```python
from build123d import *

# Parameters (mm, degrees)
SKETCH2_W           = 415
SKETCH2_H           = 210
BOSS_EXTRUDE1_DEPTH = 3
SKETCH3_W           = 415
SKETCH3_H           = 210
BOSS_EXTRUDE2_DEPTH = 3
SKETCH4_W           = 6
SKETCH4_H           = 50
SKETCH4_W_2         = 50
SKETCH4_H_2         = 6
BOSS_EXTRUDE3_DEPTH = 50
BOSS_EXTRUDE4_DEPTH = 14
SKETCH5_3_R         = 4
BOSS_EXTRUDE5_DEPTH = 350
SKETCH8_R           = 4
BOSS_EXTRUDE6_DEPTH = 14
SKETCH5_4_R         = 4
BOSS_EXTRUDE7_DEPTH = 14


with BuildPart() as part:
    # Sketch2 → Boss-Extrude1 (new body)
    with BuildSketch(Plane(origin=(0, 0, 0), x_dir=(1, 0, 0), z_dir=(0, 1, 0))):
        with Locations((207.5, 105)):
            Rectangle(SKETCH2_W, SKETCH2_H)
    extrude(amount=BOSS_EXTRUDE1_DEPTH)



with BuildPart() as body_2:
    # Sketch3 → Boss-Extrude2 (new body)
    with BuildSketch(Plane(origin=(0, 53, 0), x_dir=(1, 0, 0), z_dir=(0, 1, 0))):
        with Locations((207.5, 105)):
            Rectangle(SKETCH3_W, SKETCH3_H)
    extrude(amount=BOSS_EXTRUDE2_DEPTH)


with BuildPart() as part_1:
    add(part.part)

    add(body_2.part)  # Boss-Extrude3 merges body 2
    # Sketch4 → Boss-Extrude3 (add)
    with BuildSketch(Plane(origin=(0, 3, 0), x_dir=(1, 0, 0), z_dir=(0, 1, 0))):
        with Locations((9, 105)):
            Rectangle(SKETCH4_W, SKETCH4_H)
        with Locations((112.5, 9)):
            Rectangle(SKETCH4_W_2, SKETCH4_H_2)
        with Locations((302.5, 9)):
            Rectangle(SKETCH4_W_2, SKETCH4_H_2)
        with Locations((406, 105)):
            Rectangle(SKETCH4_W, SKETCH4_H)
        with Locations((302.5, 201)):
            Rectangle(SKETCH4_W_2, SKETCH4_H_2)
        with Locations((112.5, 201)):
            Rectangle(SKETCH4_W_2, SKETCH4_H_2)
    extrude(amount=BOSS_EXTRUDE3_DEPTH)

    # Sketch5 → Boss-Extrude4 (add)
    with BuildSketch(Plane.ZY.offset(-33.5)):
        with BuildLine():
            Line((-20.2, 66.220460186), (-20.2, 86.719329946))
            Line((-20.2, 86.719329946), (-27.7, 86.719329946))
            Line((-27.7, 86.719329946), (-27.7, 78.782856064))
            ThreePointArc((-27.7, 78.782856064), (-25, 75), (-27.7, 71.217143936))
            Line((-27.7, 71.217143936), (-27.7, 66.220460186))
            Line((-27.7, 66.220460186), (-30.3, 66.220460186))
            Line((-30.3, 66.220460186), (-30.3, 71.217143936))
            ThreePointArc((-30.3, 71.217143936), (-33, 75), (-30.3, 78.782856064))
            Line((-30.3, 78.782856064), (-30.3, 86.780809456))
            Line((-30.3, 86.780809456), (-37.8, 86.780809456))
            Line((-37.8, 86.780809456), (-37.8, 66.220460186))
            Line((-37.8, 66.220460186), (-42.5, 66.220460186))
            Line((-42.5, 66.220460186), (-42.5, 56))
            Line((-42.5, 56), (-15.5, 56))
            Line((-15.5, 56), (-15.5, 66.220460186))
            Line((-15.5, 66.220460186), (-20.2, 66.220460186))
        make_face()
        with BuildLine():
            Line((-149.888097116, 72.9128735), (-155.8, 72.9128735))
            Line((-155.8, 72.9128735), (-155.8, 56))
            Line((-155.8, 56), (-125.8, 56))
            Line((-125.8, 56), (-125.8, 72.9128735))
            Line((-125.8, 72.9128735), (-131.711902884, 72.9128735))
            ThreePointArc((-131.711902884, 72.9128735), (-140.8, 93.165324665), (-149.888097116, 72.9128735))
        make_face()
    extrude(amount=-BOSS_EXTRUDE4_DEPTH)

    # Sketch5_3 → Boss-Extrude5 (add)
    with BuildSketch(Plane.ZY.offset(-33.5)):
        with Locations((-140.8, 81)):
            Circle(SKETCH5_3_R)
        with BuildLine():
            Line((-30.3, 71.217143936), (-30.3, 78.782856064))
            ThreePointArc((-30.3, 78.782856064), (-33, 75), (-30.3, 71.217143936))
        make_face()
        with BuildLine():
            Line((-27.7, 71.217143936), (-27.7, 78.782856064))
            ThreePointArc((-27.7, 78.782856064), (-29, 79), (-30.3, 78.782856064))
            Line((-30.3, 78.782856064), (-30.3, 71.217143936))
            ThreePointArc((-30.3, 71.217143936), (-29, 71), (-27.7, 71.217143936))
        make_face()
        with BuildLine():
            ThreePointArc((-25, 75), (-25.744235881, 77.323790008), (-27.7, 78.782856064))
            Line((-27.7, 78.782856064), (-27.7, 71.217143936))
            ThreePointArc((-27.7, 71.217143936), (-25.744235881, 72.676209992), (-25, 75))
        make_face()
    extrude(amount=-BOSS_EXTRUDE5_DEPTH)

    # Sketch8 → Boss-Extrude6 (add)
    with BuildSketch(Plane(origin=(361, 0, 0), x_dir=(0, 0, -1), z_dir=(1, 0, 0))):
        with BuildLine():
            Line((37.8, 66.220460186), (37.8, 86.719329946))
            Line((37.8, 86.719329946), (30.3, 86.719329946))
            Line((30.3, 86.719329946), (30.3, 78.782856064))
            ThreePointArc((30.3, 78.782856064), (33, 75), (30.3, 71.217143936))
            Line((30.3, 71.217143936), (30.3, 66.220460186))
            Line((30.3, 66.220460186), (27.7, 66.220460186))
            Line((27.7, 66.220460186), (27.7, 71.217143936))
            ThreePointArc((27.7, 71.217143936), (25, 75), (27.7, 78.782856064))
            Line((27.7, 78.782856064), (27.7, 86.780809456))
            Line((27.7, 86.780809456), (20.2, 86.780809456))
            Line((20.2, 86.780809456), (20.2, 66.220460186))
            Line((20.2, 66.220460186), (15.5, 66.220460186))
            Line((15.5, 66.220460186), (15.5, 56))
            Line((15.5, 56), (42.5, 56))
            Line((42.5, 56), (42.5, 66.220460186))
            Line((42.5, 66.220460186), (37.8, 66.220460186))
        make_face()
        with BuildLine():
            Line((131.711902884, 72.9128735), (125.8, 72.9128735))
            Line((125.8, 72.9128735), (125.8, 56))
            Line((125.8, 56), (155.8, 56))
            Line((155.8, 56), (155.8, 72.9128735))
            Line((155.8, 72.9128735), (149.888097116, 72.9128735))
            ThreePointArc((149.888097116, 72.9128735), (140.8, 93.165324665), (131.711902884, 72.9128735))
        make_face()
        with Locations((140.8, 81)):
            Circle(SKETCH8_R, mode=Mode.SUBTRACT)
    extrude(amount=BOSS_EXTRUDE6_DEPTH)

    # Sketch5_4 → Boss-Extrude7 (add)
    with BuildSketch(Plane.ZY.offset(-33.5)):
        with Locations((-140.8, 81)):
            Circle(SKETCH5_4_R)
        with BuildLine():
            ThreePointArc((-25, 75), (-25.744235881, 77.323790008), (-27.7, 78.782856064))
            Line((-27.7, 78.782856064), (-27.7, 71.217143936))
            ThreePointArc((-27.7, 71.217143936), (-25.744235881, 72.676209992), (-25, 75))
        make_face()
        with BuildLine():
            Line((-27.7, 71.217143936), (-27.7, 78.782856064))
            ThreePointArc((-27.7, 78.782856064), (-29, 79), (-30.3, 78.782856064))
            Line((-30.3, 78.782856064), (-30.3, 71.217143936))
            ThreePointArc((-30.3, 71.217143936), (-29, 71), (-27.7, 71.217143936))
        make_face()
        with BuildLine():
            Line((-30.3, 71.217143936), (-30.3, 78.782856064))
            ThreePointArc((-30.3, 78.782856064), (-33, 75), (-30.3, 71.217143936))
        make_face()
    extrude(amount=BOSS_EXTRUDE7_DEPTH)


solid = part_1.part
```
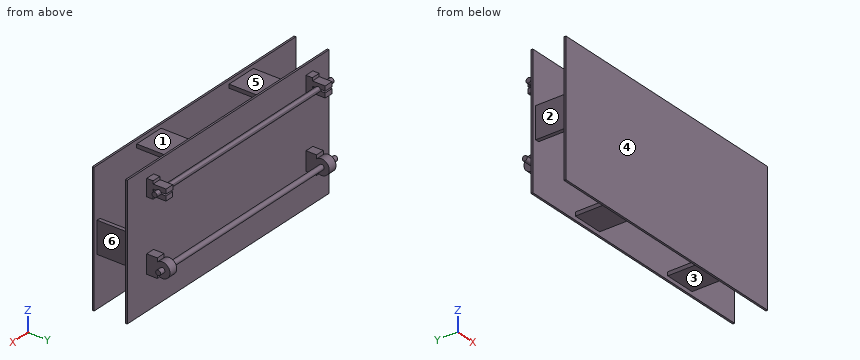
Source: CAD feature listing. Evaluate the final solid. Frame: model axes, mm. Face numbers are marked on the shaded views. A direction names the side the tool comes from. Round coordinates to 2 decimals unless told otherwise and drop trailing zeros. Loops run counter-clockwise (first coordinate to the right, second up) from the corner with the lowest first, then second, coordinate; pieces in that order, holes last. Notation, with made-up numbers: M 80,-19 L 101,-19 A11 ccw 101,-1 Z; hole C -10,42 d3. An arc over 180 degrees is marked long. Use a Markdown table: item, result. Add a question column.
1. Ray query, line 1 along Y through (x, z) = (236.5, -141) (3 decimals); line 2 along X through (y, z) = (12, -94.5); line 3 along X through (y, z) = (82.5, -149.5). Return the intervals inside material, ascending. Write a range as [from, to].
2. Cut plane A-A, the plane z = -161. Output: boundary loops of the cut face in (x, y), and give its area (3 significant figures).
3. Cut plane C-C, the plane y = 38. Output: boundary loops of the cut face in (x, z), and give its area (3 significant figures).
4. Cut plane B-B, the plane x = 248. Output: boundary loops of the cut face in (y, z), and give its area (3 significant figures).
5. Pull-direction query (Y, two-part tool) for the marked faces 4, 5 and 6; classes: +Y half, -Y half, draft (parallel to the pull), parting line (faces both ways), or undercut.
6. Contact query for flat-ended pins moving along their axis: pin 1 (10 mm diameter, centred on x = 150.5, z = -131, fed in from -Y); pin 2 (0.8 mm diameter, centred on x = 367, z = -29, fed in from +Y); pin 3 (1.8 mm diameter, centred on y = 33, z = -8.5, fed in from -X); pin 4 (21.5 mm diameter, centred on y = 76.5, z = -23.5, fed in from -X). Output: stop coordinate, or through.
7. Cut plane D-D, the plane y = 62. Output: boundary loops of the cut face in (x, z), and give its area (3 significant figures).
8. Set-up query: the marked faces 1, 2 and 3. Return all of +Z, -Z, +X, -X, +Y, -Y with unobstructed straight access to the full face (end or side cutting, diameter ignored); none if empty.
Solution:
| question | item | result |
|---|---|---|
| 1 | line 1 | y = [0, 3], [53, 56], [77.005, 84.995] |
| 1 | line 2 | x = [6, 12], [403, 409] |
| 1 | line 3 | x = [33.5, 47.5], [361, 375] |
| 2 | outline | M 0,0 L 415,0 L 415,3 L 0,3 Z; M 0,53 L 415,53 L 415,56 L 0,56 Z |
| 2 | area | 2,490 mm2 |
| 3 | outline | M 6,-130 L 12,-130 L 12,-80 L 6,-80 Z; M 87.5,-204 L 137.5,-204 L 137.5,-198 L 87.5,-198 Z; M 87.5,-12 L 137.5,-12 L 137.5,-6 L 87.5,-6 Z; M 277.5,-204 L 327.5,-204 L 327.5,-198 L 277.5,-198 Z; M 277.5,-12 L 327.5,-12 L 327.5,-6 L 277.5,-6 Z; M 403,-130 L 409,-130 L 409,-80 L 403,-80 Z |
| 3 | area | 1,800 mm2 |
| 4 | outline | M 0,-210 L 3,-210 L 3,0 L 0,0 Z; M 53,-210 L 56,-210 L 56,0 L 53,0 Z; C 75,-29 d8; C 81,-140.8 d8 |
| 4 | area | 1,360 mm2 |
| 5 | face 4 | -Y half |
| 5 | face 5 | undercut |
| 5 | face 6 | undercut |
| 6 | pin 1 | stops at y = 0 |
| 6 | pin 2 | stops at y = 79 |
| 6 | pin 3 | stops at x = 87.5 |
| 6 | pin 4 | stops at x = 19.5 |
| 7 | outline | M 33.5,-155.8 L 47.5,-155.8 L 47.5,-125.8 L 33.5,-125.8 Z; M 33.5,-42.5 L 47.5,-42.5 L 47.5,-15.5 L 33.5,-15.5 Z; M 361,-155.8 L 375,-155.8 L 375,-125.8 L 361,-125.8 Z; M 361,-42.5 L 375,-42.5 L 375,-15.5 L 361,-15.5 Z |
| 7 | area | 1,600 mm2 |
| 8 | face 1 | +Z, +X, -X |
| 8 | face 2 | +Z, -Z, -X |
| 8 | face 3 | -Z, +X, -X |
